Geometry: final body of the model. Coordinates: model frame, mm. A direction names the side the tool comes from. Give positions to 0.01 mm unless a question says otherwise; leave off trailing zeros. Loops run counter-clockwise (first coordinate to the right, second up) from the corner with the lowest first, then second, coordinate; pieces in that order, holes last.
from build123d import *

# Parameters (mm, degrees)
PAD_DEPTH       = 6
PAD001_DEPTH    = 2
SKETCH002_R     = 1.6
POCKET_DEPTH    = 8.001
POCKET001_DEPTH = 4
FILLET_R        = 4
FILLET001_R     = 1


with BuildPart() as part:
    # Sketch → Pad (new body)
    with BuildSketch(Plane.XY):
        with BuildLine():
            Line((32.5, 18), (32.5, -12))
            Line((32.5, -12), (-32.5, -12))
            Line((-32.5, -12), (-32.5, 18))
            Line((-32.5, 18), (-13.856406, 18))
            ThreePointArc((13.856406, 18), (0, 26), (-13.856406, 18))
            Line((32.5, 18), (13.856406, 18))
        make_face()
        with BuildLine():
            ThreePointArc((22.9, -5), (25, -7.1), (27.1, -5))
            Line((27.1, -5), (27.1, 6))
            ThreePointArc((27.1, 6), (25, 8.1), (22.9, 6))
            Line((22.9, -5), (22.9, 6))
        make_face(mode=Mode.SUBTRACT)
        with BuildLine():
            ThreePointArc((-27.1, -5), (-25, -7.1), (-22.9, -5))
            Line((-22.9, -5), (-22.9, 6))
            ThreePointArc((-22.9, 6), (-25, 8.1), (-27.1, 6))
            Line((-27.1, -5), (-27.1, 6))
        make_face(mode=Mode.SUBTRACT)
    extrude(amount=PAD_DEPTH)

    # Sketch001 → Pad001 (new body)
    with BuildSketch(Plane.XY.offset(6)):
        with BuildLine():
            Line((5, -12), (-5, -12))
            Line((-5, -12), (-5, 4))
            ThreePointArc((-17.5, 4.829723), (-11.257647, 4.299661), (-5, 4))
            Line((-17.5, 4.829723), (-17.5, 9.829723))
            ThreePointArc((-17.5, 9.829723), (0, 8.899068), (17.5, 9.829723))
            Line((17.5, 4.829723), (17.5, 9.829723))
            ThreePointArc((5, 4), (11.257647, 4.299661), (17.5, 4.829723))
            Line((5, -12), (5, 4))
        make_face()
    extrude(amount=PAD001_DEPTH)

    # Sketch002 → Pocket (cut, through all)
    with BuildSketch(Plane.XY.offset(8)):
        with Locations((0, 2)):
            Circle(SKETCH002_R)
    extrude(amount=-POCKET_DEPTH, mode=Mode.SUBTRACT)

    # Sketch003 → Pocket001 (cut)
    with BuildSketch(Plane(origin=(0, 0, 0), x_dir=(1, 0, 0), z_dir=(0, 0, -1))):
        Polygon((2.85, -3.645448), (2.85, -0.354552), (0, 1.290897), (-2.85, -0.354552), (-2.85, -3.645448), (0, -5.290897), align=None)
    extrude(amount=-POCKET001_DEPTH, mode=Mode.SUBTRACT)

    # Fillet
    fillet_edges = [part.edges().sort_by_distance(p)[0] for p in [
        (32.5, 18, 3),
        (32.5, -12, 3),
        (-32.5, 18, 3),
        (-32.5, -12, 3),
    ]]
    fillet(fillet_edges, radius=FILLET_R)

    # Fillet001
    fillet001_edges = [part.edges().sort_by_distance(p)[0] for p in [
        (17.5, 9.829723, 7),
        (17.5, 4.829723, 7),
        (-17.5, 9.829723, 7),
        (-17.5, 4.829723, 7),
        (-13.856406, 18, 3),
        (13.856406, 18, 3),
    ]]
    fillet(fillet001_edges, radius=FILLET001_R)


solid = part.part
Item 1: Section query B-B on x = -25. Return loops of the section in (y, z), plus the area to 3 significant figures.
Values follow:
outline: (-12, 0) - (-7.1, 0) - (-7.1, 6) - (-12, 6) - close; (8.1, 0) - (18, 0) - (18, 6) - (8.1, 6) - close
area: 88.8 mm2
Item 2: Section query C-C on z = 7. Return loops of the section in (x, y), plus the area to 3 significant figures.
Values follow:
outline: (-17.5, 5.73) arc R1 ccw to (-16.6, 4.74) arc R169.97 ccw to (-5, 4) - (-5, -12) - (5, -12) - (5, 4) arc R169.97 ccw to (16.6, 4.74) arc R1 ccw to (17.5, 5.73) - (17.5, 8.72) arc R1 ccw to (16.4, 9.72) arc R165 cw to (-16.4, 9.72) arc R1 ccw to (-17.5, 8.72) - close; hole circle Ø3.2 at (0, 2)
area: 325 mm2
Item 3: Set-up query: faces 4 (the face through (-0.2, 8.9, 7)), 5 (the face through (25, -7.1, 3)), 6 (the face through (-17.5, 7, 7)), 7 (the face through (1.405, 4.48, 1.972)), 8 (the face through (22, 18, 3)). Return all of +Z, -Z, +X, -X, +Y, -Y with unobstructed straight access to the full face (end or side cutting, diameter ignored); none if empty.
Values follow:
face 4: +Z, +Y
face 5: +Z, -Z
face 6: +Z, -X, +Y, -Y
face 7: -Z
face 8: +Z, -Z, +X, +Y
Item 4: Section query D-D on z = 2.5. Return loops of the section in (x, y), plus the area to 3 significant figures.
Values follow:
outline: (-32.5, -8) arc R4 ccw to (-28.5, -12) - (28.5, -12) arc R4 ccw to (32.5, -8) - (32.5, 14) arc R4 ccw to (28.5, 18) - (14.42, 18) arc R1 cw to (13.57, 18.47) arc R16 ccw to (-13.57, 18.47) arc R1 cw to (-14.42, 18) - (-28.5, 18) arc R4 ccw to (-32.5, 14) - close; hole (-27.1, -5) arc R2.1 ccw to (-22.9, -5) - (-22.9, 6) arc R2.1 ccw to (-27.1, 6) - close; hole (-2.85, 0.35) - (0, -1.29) - (2.85, 0.35) - (2.85, 3.65) - (0, 5.29) - (-2.85, 3.65) - close; hole (22.9, -5) arc R2.1 ccw to (27.1, -5) - (27.1, 6) arc R2.1 ccw to (22.9, 6) - close
area: 1,950 mm2
Item 5: Draft query along X for faces 1 (the face through (-32.5, 3, 3)), 2 (the face through (-25, -7.1, 3)), 3 (the face through (-22, 18, 3)). Return one class per face: +X half, -X half, draft (parallel to the pull), parting line (faces both ways), or undercut.
Values follow:
face 1: -X half
face 2: undercut
face 3: draft
Item 6: Ray query, probe 1 along X at (y, z) = (-4, 5.25); probe 2 along Y at (x, z) = (0, 6.05); probe 3 along Y at (x, z) = (0, 5.9). Return the intervals inside material, ascending.
Values follow:
probe 1: x = -32.5 to -27.1, -22.9 to 22.9, 27.1 to 32.5
probe 2: y = -12 to 0.4, 3.6 to 8.9
probe 3: y = -12 to 0.4, 3.6 to 26
Item 7: Pin query (flat end, axial travel): pin 1 (1 mm diameter, centred on y = -7, z = 7, fed in from -X); pin 2 (1 mm diameter, centred on x = -22, y = -6, fed in from +Z); pin 3 (1.9 mm diameter, centred on x = 0, y = 2, fed in from -Z); pin 4 (1 mm diameter, centred on y = 7, z = 7, fed in from +X). Return the tip coordinate at first contact, or that it passes through.
Values follow:
pin 1: stops at x = -5
pin 2: stops at z = 6
pin 3: passes through
pin 4: stops at x = 17.5
Item 8: Section query A-A on y = 2. Return loops of the section in (x, z).
Values follow:
outline: (-32.5, 0) - (-27.1, 0) - (-27.1, 6) - (-32.5, 6) - close; (-22.9, 0) - (-2.85, 0) - (-2.85, 4) - (-1.6, 4) - (-1.6, 8) - (-5, 8) - (-5, 6) - (-22.9, 6) - close; (1.6, 4) - (2.85, 4) - (2.85, 0) - (22.9, 0) - (22.9, 6) - (5, 6) - (5, 8) - (1.6, 8) - close; (27.1, 0) - (32.5, 0) - (32.5, 6) - (27.1, 6) - close
